from build123d import *

# Parameters (mm, degrees)
F0_W     = 76.2
F0_H     = 76.2
F0_R     = 2.032
F1_DEPTH = 0.8128
F2_R     = 6.35


with BuildPart() as f1:
    # F0 (on Top) → F1 (new body)
    with BuildSketch(Plane.XY):
        Rectangle(F0_W, F0_H)
        with Locations((-31.75, -31.75)):
            Circle(F0_R, mode=Mode.SUBTRACT)
        with Locations((-19.05, -31.75)):
            Circle(F0_R, mode=Mode.SUBTRACT)
        with Locations((-6.35, -31.75)):
            Circle(F0_R, mode=Mode.SUBTRACT)
        with Locations((-31.75, -19.05)):
            Circle(F0_R, mode=Mode.SUBTRACT)
        with Locations((-31.75, -6.35)):
            Circle(F0_R, mode=Mode.SUBTRACT)
        with Locations((-19.05, -19.05)):
            Circle(F0_R, mode=Mode.SUBTRACT)
        with Locations((-6.35, -19.05)):
            Circle(F0_R, mode=Mode.SUBTRACT)
        with Locations((-19.05, -6.35)):
            Circle(F0_R, mode=Mode.SUBTRACT)
        with Locations((-6.35, -6.35)):
            Circle(F0_R, mode=Mode.SUBTRACT)
        with Locations((6.35, -31.75)):
            Circle(F0_R, mode=Mode.SUBTRACT)
        with Locations((19.05, -31.75)):
            Circle(F0_R, mode=Mode.SUBTRACT)
        with Locations((31.75, -31.75)):
            Circle(F0_R, mode=Mode.SUBTRACT)
        with Locations((6.35, -19.05)):
            Circle(F0_R, mode=Mode.SUBTRACT)
        with Locations((6.35, -6.35)):
            Circle(F0_R, mode=Mode.SUBTRACT)
        with Locations((19.05, -19.05)):
            Circle(F0_R, mode=Mode.SUBTRACT)
        with Locations((31.75, -19.05)):
            Circle(F0_R, mode=Mode.SUBTRACT)
        with Locations((19.05, -6.35)):
            Circle(F0_R, mode=Mode.SUBTRACT)
        with Locations((31.75, -6.35)):
            Circle(F0_R, mode=Mode.SUBTRACT)
        with Locations((-31.75, 6.35)):
            Circle(F0_R, mode=Mode.SUBTRACT)
        with Locations((-19.05, 6.35)):
            Circle(F0_R, mode=Mode.SUBTRACT)
        with Locations((-6.35, 6.35)):
            Circle(F0_R, mode=Mode.SUBTRACT)
        with Locations((-31.75, 19.05)):
            Circle(F0_R, mode=Mode.SUBTRACT)
        with Locations((-31.75, 31.75)):
            Circle(F0_R, mode=Mode.SUBTRACT)
        with Locations((-19.05, 19.05)):
            Circle(F0_R, mode=Mode.SUBTRACT)
        with Locations((-6.35, 19.05)):
            Circle(F0_R, mode=Mode.SUBTRACT)
        with Locations((-19.05, 31.75)):
            Circle(F0_R, mode=Mode.SUBTRACT)
        with Locations((-6.35, 31.75)):
            Circle(F0_R, mode=Mode.SUBTRACT)
        with Locations((6.35, 6.35)):
            Circle(F0_R, mode=Mode.SUBTRACT)
        with Locations((19.05, 6.35)):
            Circle(F0_R, mode=Mode.SUBTRACT)
        with Locations((31.75, 6.35)):
            Circle(F0_R, mode=Mode.SUBTRACT)
        with Locations((6.35, 19.05)):
            Circle(F0_R, mode=Mode.SUBTRACT)
        with Locations((6.35, 31.75)):
            Circle(F0_R, mode=Mode.SUBTRACT)
        with Locations((19.05, 19.05)):
            Circle(F0_R, mode=Mode.SUBTRACT)
        with Locations((31.75, 19.05)):
            Circle(F0_R, mode=Mode.SUBTRACT)
        with Locations((19.05, 31.75)):
            Circle(F0_R, mode=Mode.SUBTRACT)
        with Locations((31.75, 31.75)):
            Circle(F0_R, mode=Mode.SUBTRACT)
    extrude(amount=F1_DEPTH)

    # F2
    f2_edges = [f1.edges().sort_by_distance(p)[0] for p in [
        (-38.1, -38.1, 0.4064),
        (38.1, -38.1, 0.4064),
        (38.1, 38.1, 0.4064),
        (-38.1, 38.1, 0.4064),
    ]]
    fillet(f2_edges, radius=F2_R)


solid = f1.part
The model under review builds one solid part; all positions refer to its coordinate system, in mm. Give positions to 0.01 mm unless a question says otherwise; leave off trailing zeros. Order: outer loops, then holes, each group sorted by start corner. A loop starts at its lowest first (then second) coordinate and runs counter-clockwise, first axis right, second up. Notation, with made-up numbers: M 18.25,72.5 L 72.25,72.5 A17 ccw 72.25,83.5 Z; hole C 26,16 d4. An arc over 180 degrees is marked long. Answer in a Markdown table with one row per item. Add a question column.
1. Add section A-A on x = 19.05. State the section outline as (y, z) points.
2. For pin 1 Ø2.5 at (x, y) = (-19.05, 6.35) entering from -Z, flat-tipped, find the tip position at first contact; note if it passes through.
3. Mouldability with a two-part tool opening along Y and no side actions: class faces 1 (the cylindrical face through (-36.29, 36.19, 0.41)), 2 (the cylindrical face through (-17.958, -17.337, 0.401)) as released by +Y, released by -Y, zero draft, split by the parting line, or undercut.
4. Add section C-C on z = 0.5. Count the separate pieces of the cut face and the enclosed holes in it, plus the area to 3 significant figures.
The answers:
| question | item | result |
|---|---|---|
| 1 | outline | M -38.1,0 L -33.78,0 L -33.78,0.81 L -38.1,0.81 Z; M -29.72,0 L -21.08,0 L -21.08,0.81 L -29.72,0.81 Z; M -17.02,0 L -8.38,0 L -8.38,0.81 L -17.02,0.81 Z; M -4.32,0 L 4.32,0 L 4.32,0.81 L -4.32,0.81 Z; M 8.38,0 L 17.02,0 L 17.02,0.81 L 8.38,0.81 Z; M 21.08,0 L 29.72,0 L 29.72,0.81 L 21.08,0.81 Z; M 33.78,0 L 38.1,0 L 38.1,0.81 L 33.78,0.81 Z |
| 2 | pin 1 | through |
| 3 | face 1 | released by +Y |
| 3 | face 2 | undercut |
| 4 | separate pieces | 1 |
| 4 | enclosed holes | 36 |
| 4 | area | 5,300 mm2 |
